Geometry: final body of the model. Coordinates: model frame, mm. Face numbers are marked on the shaded views. A direction names the side the tool comes from. Round coordinates to 2 decimals unless told otherwise and drop trailing zeros. Write each loop counter-clockwise with the first axis right and the second up, starting at its lowest first coordinate (ties: lowest second). Pieces come first, ordered by that corner, then holes. Notation, with made-up numbers: (59.5, -5) - (93.5, -5) arc R21 ccw to (93.5, 12) - close; hole circle Ø11 at (-37, 80.25). An arc over 180 degrees is marked (long way). Write each question's results on one line, items separated by ' | '.
from build123d import *

# Parameters (mm, degrees)
ESQUISSE1_W             = 70
ESQUISSE1_H             = 20
BOSS_EXTRU_1_DEPTH      = 5
ESQUISSE2_W             = 70
ESQUISSE2_H             = 5
BOSS_EXTRU_2_DEPTH      = 70
ESQUISSE3_R             = 1.5
ENL_V_MAT_EXTRU_1_DEPTH = 60


with BuildPart() as part:
    # Esquisse1 → Boss.-Extru.1 (new body)
    with BuildSketch(Plane.XY):
        with Locations((-35, 10)):
            Rectangle(ESQUISSE1_W, ESQUISSE1_H)
    extrude(amount=BOSS_EXTRU_1_DEPTH)

    # Esquisse2 → Boss.-Extru.2 (add)
    with BuildSketch(Plane.XY.offset(5)):
        with Locations((-35, 17.5)):
            Rectangle(ESQUISSE2_W, ESQUISSE2_H)
    extrude(amount=BOSS_EXTRU_2_DEPTH)

    # Esquisse3 → Enlèv. mat.-Extru.1 (cut)
    with BuildSketch(Plane(origin=(0, 0, 0), x_dir=(-1, 0, 0), z_dir=(0, 0, -1))):
        with Locations((35, 3.26755804)):
            Circle(ESQUISSE3_R)
    extrude(amount=-ENL_V_MAT_EXTRU_1_DEPTH, mode=Mode.SUBTRACT)


solid = part.part
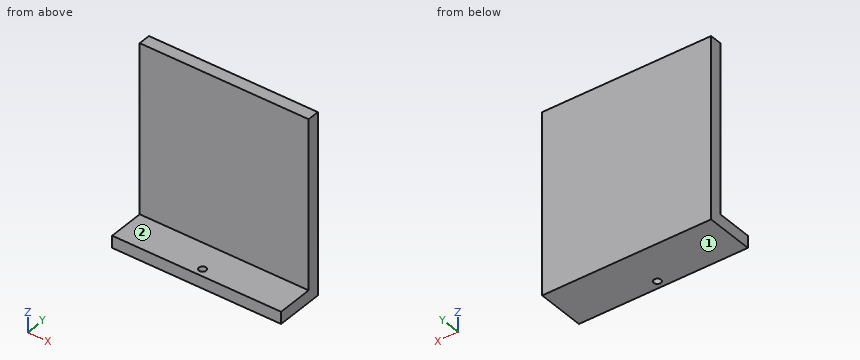
Q1. Section query A-A, the plane x = -35. Return loops of the section in (y, z).
Answer block:
outline: (0, 0) - (1.77, 0) - (1.77, 5) - (0, 5) - close; (4.77, 0) - (20, 0) - (20, 75) - (15, 75) - (15, 5) - (4.77, 5) - close
Q2. Section query D-D, the plane y = 6. Return loops of the section in (x, z).
Answer block:
outline: (-70, 0) - (0, 0) - (0, 5) - (-70, 5) - close
Q3. Ray query, line 1 along Y through (x, z) = (-35, 3); line 2 along Y through (x, z) = (-11.5, 41); line 3 along Z through (x, y) = (-33, 13.5). Return the intervals inside material, ascending.
Answer block:
line 1: 0 to 1.77, 4.77 to 20 | line 2: 15 to 20 | line 3: 0 to 5
Q4. Pin query (flat end, axial travel): pin 1 (7.5 mm diameter, centred on x = -26, y = 6, fed in from +Z); pin 2 (21 mm diameter, centred on x = -33.5, z = 56.5, fed in from -Y). Return the tip coordinate at first contact, or that it passes through.
Answer block:
pin 1: z = 5 | pin 2: y = 15
Q5. Section query B-B, the plane x = -12.5. Return loops of the section in (y, z).
Answer block:
outline: (0, 0) - (20, 0) - (20, 75) - (15, 75) - (15, 5) - (0, 5) - close
Q6. Access query for the marked faces 1 and 2. Directions: +Z, -Z, +X, -X, +Y, -Y. A direction counts if a zero-diameter tool reaches every point of the face in a straight line with its end or side. Return the directions, or none.
Answer block:
face 1: -Z, +X, -X, +Y, -Y | face 2: +Z, +X, -X, -Y
Q7. Section query C-C, the plane z = 38.5. Return loops of the section in (x, y), plus the area to 3 significant figures.
Answer block:
outline: (-70, 15) - (0, 15) - (0, 20) - (-70, 20) - close | area: 350 mm2
